Answer from the drawing. Dimensions are ordinates in mm from the lowest x, y and z of the part. Round coordinates to 2 decimals unless told otherwise and drop trailing zeros. Order: outer loops, then holes, each group sorted by start corner. A loop starts at its lowest first (then second) coordinate and runs counter-clockwise, first axis right, second up. Notation, with made-up numbers: M -26.75,66.25 L -10.75,66.25 A25 ccw -10.75,80.25 Z; hole C 35,-29.75 d11. An arc over 180 degrees is marked long. Answer as a JSON object with one key per item and string values. Group by question number.
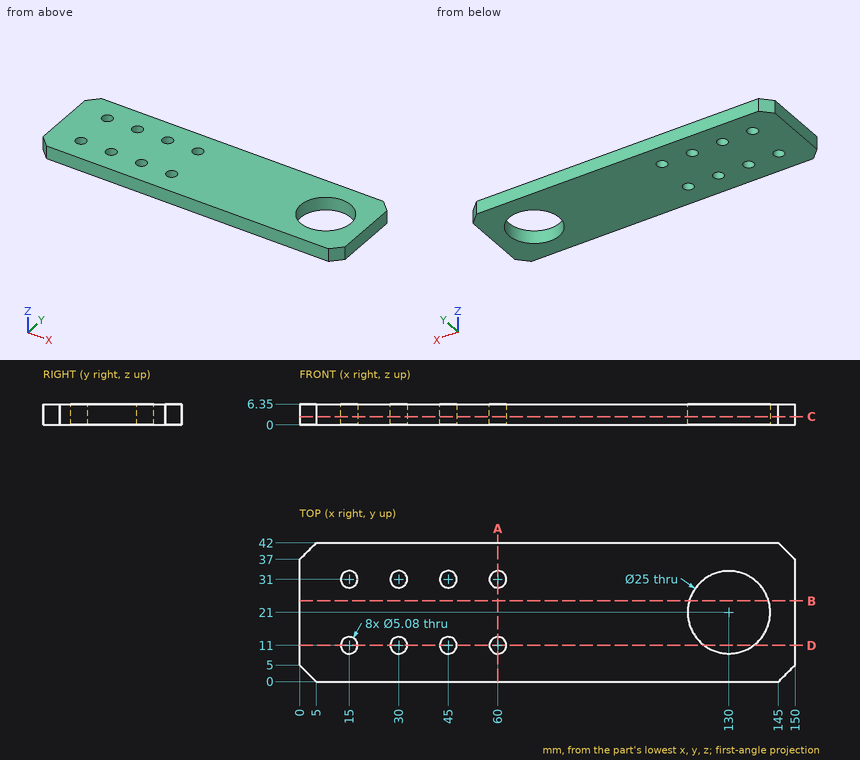
Item 1: Find section A-A (x = 60). Give the vertices of the cut face in (y, z), and give its area (3 significant figures).
Item 2: This flat-tipped pin is pushed along its axis until it touches: pin 1 (3 mm diameter, centred on x = 15, y = 11, fed in from +Z). Where does it stop, or does it pass through?
Item 3: Consider L1, parallel to Y at x = 15, z = 5; L2, parallel to X at y = 20.5, z = 2.5; L3, parallel to Y at x = 16.5, z = 6. Determine where each line is inside the solid, lowest interval first.
Item 4: Find section B-B (y = 24.5). Give the vertices of the cut face in (x, z).
Item 5: Find section C-C (z = 2.5). Give the number of separate pieces and of enclosed holes in the cut face, and give its area (3 significant figures).
Item 6: Find section D-D (y = 11). Give the vertices of the cut face in (x, z).
Responses:
{
 "1": {"outline": "M 0,0 L 8.46,0 L 8.46,6.35 L 0,6.35 Z; M 13.54,0 L 28.46,0 L 28.46,6.35 L 13.54,6.35 Z; M 33.54,0 L 42,0 L 42,6.35 L 33.54,6.35 Z", "area": "202 mm^2"},
 "2": {"pin 1": "passes through"},
 "3": {"L1": "y = 0 to 8.46, 13.54 to 28.46, 33.54 to 42", "L2": "x = 0 to 117.51, 142.49 to 150", "L3": "y = 0 to 8.95, 13.05 to 28.95, 33.05 to 42"},
 "4": {"outline": "M 0,0 L 118,0 L 118,6.35 L 0,6.35 Z; M 142,0 L 150,0 L 150,6.35 L 142,6.35 Z"},
 "5": {"separate pieces": "1", "enclosed holes": "9", "area": "5,600 mm^2"},
 "6": {"outline": "M 0,0 L 12.46,0 L 12.46,6.35 L 0,6.35 Z; M 17.54,0 L 27.46,0 L 27.46,6.35 L 17.54,6.35 Z; M 32.54,0 L 42.46,0 L 42.46,6.35 L 32.54,6.35 Z; M 47.54,0 L 57.46,0 L 57.46,6.35 L 47.54,6.35 Z; M 62.54,0 L 122.5,0 L 122.5,6.35 L 62.54,6.35 Z; M 137.5,0 L 150,0 L 150,6.35 L 137.5,6.35 Z"}
}
